Source: CAD feature listing. Evaluate the final solid. Frame: model axes, mm. Face numbers are marked on the shaded views. A direction names the side the tool comes from. Coordinates: 2 decimals unless noted, no trailing zeros. Write each loop counter-clockwise with the first axis right and the second up, starting at its lowest first coordinate (ties: lowest second). Pieces come first, ordered by that corner, then holes. Notation, with made-up numbers: (16.25, -39.5) - (48.25, -39.5) arc R17 cw to (48.25, -33.5) - close; hole circle Ø10 at (-22.75, -40). An arc over 180 degrees is marked (long way). One line per question, with ' | ' between items. Start each with the question number.
Q1. Access query for the marked faces 4 and 5. Directions: +Z, -Z, +X, -X, +Y, -Y. A direction counts if a zero-diameter tool reaches every point of the face in a straight line with its end or side. Return the directions, or none.
Q2. Draft query along X for the marked faces 1, 2 and 3. Return one class per face: +X half, -X half, draft (parallel to the pull), parting line (faces both ways), or undercut.
Q3. Cut plane A-A, the plane z = 3.2. Return loops of the section in (x, y) (3 decimals), plus the area to 3 significant figures.
Q4. Line query: line 1 (X direction, y = -63.15, z = 3.2); line 2 (Z direction, x = -11, y = -63.25); line 3 (Y direction, x = 0, z = 5.75). Output: solid intervals per line, ascending.
Q5. Cut plane C-C, the plane z = 5.5. Return loops of the section in (x, y) (3 decimals), plus the area to 3 significant figures.
Q6. Cut plane B-B, the plane x = -10.5. Return loops of the section in (y, z).
Q7. Contact query for flat-ended pins moving along their axis: P1, Ø2, axis at x = 5.5, z = 4.5, coming from the +Y side (3 decimals); P2, Ø3, axis at x = -10, z = 2, coming from the +Y side; P3, Ø2, axis at y = -54, z = 4, coming from the +X side. Output: stop coordinate, or through.
Q8. Cut plane D-D, the plane y = -40. Return loops of the section in (x, z), plus the area to 3 significant figures.
```python
from build123d import *

# Parameters (mm, degrees)
BOSS_EXTRUDE1_DEPTH = 6
SKETCH2_R           = 1.6
CUT_EXTRUDE1_DEPTH  = 10
FILLET1_R           = 1


with BuildPart() as part:
    # Sketch1 → Boss-Extrude1 (new body)
    with BuildSketch(Plane.XY):
        with BuildLine():
            Line((-6.342263295, -37.122659043), (-7.672233378, -62.5))
            Line((-7.672233378, -62.5), (-14, -62.5))
            Line((-14, -62.5), (-14, -65.5))
            Line((-14, -65.5), (14, -65.5))
            Line((14, -65.5), (14, -62.5))
            Line((14, -62.5), (7.672233378, -62.5))
            Line((7.672233378, -62.5), (6.342263295, -37.122659043))
            ThreePointArc((6.342263295, -37.122659043), (5.670701308, -36.229994036), (4.591009287, -36.516544999))
            ThreePointArc((4.591009287, -36.516544999), (0, -38.6), (-4.591009287, -36.516544999))
            ThreePointArc((-4.591009287, -36.516544999), (-5.670701308, -36.229994036), (-6.342263295, -37.122659043))
        make_face()
    extrude(amount=BOSS_EXTRUDE1_DEPTH)

    # Sketch2 → Cut-Extrude1 (cut)
    with BuildSketch(Plane.XZ.offset(65.5)):
        with Locations(Location((10.872233378, 3.2, 0), (0, 0, 270))):
            Circle(SKETCH2_R)
        with Locations(Location((-10.872233378, 3.2, 0), (0, 0, 270))):
            Circle(SKETCH2_R)
    extrude(amount=-CUT_EXTRUDE1_DEPTH, mode=Mode.SUBTRACT)

    # Fillet1
    fillet1_edges = [part.edges().sort_by_distance(p)[0] for p in [
        (-14, -64, 6),
        (14, -64, 6),
    ]]
    fillet(fillet1_edges, radius=FILLET1_R)


solid = part.part
```
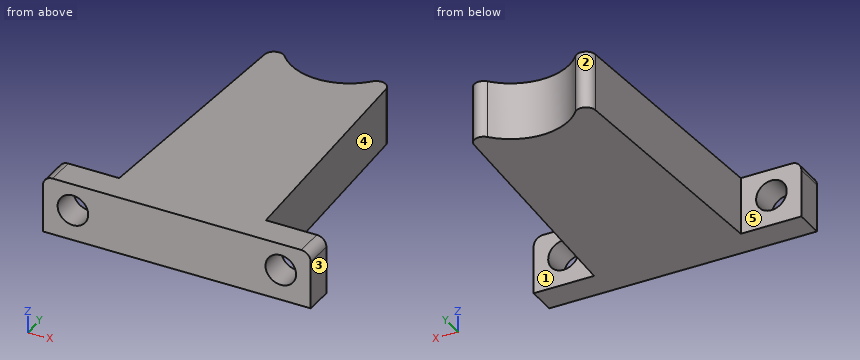
Reply:
1) face 4: +Z, -Z, +X, +Y | face 5: +Z, -Z, -X, +Y
2) face 1: draft | face 2: undercut | face 3: +X half
3) outline: (-14, -65.5) - (-12.472, -65.5) - (-12.472, -62.5) - (-14, -62.5) - close; (-9.272, -65.5) - (9.272, -65.5) - (9.272, -62.5) - (7.672, -62.5) - (6.342, -37.123) arc R1 ccw to (4.591, -36.517) arc R6.1 cw to (-4.591, -36.517) arc R1 ccw to (-6.342, -37.123) - (-7.672, -62.5) - (-9.272, -62.5) - close; (12.472, -65.5) - (14, -65.5) - (14, -62.5) - (12.472, -62.5) - close | area: 415 mm^2
4) line 1: x = -14 to -12.47, -9.27 to 9.27, 12.47 to 14 | line 2: z = 0 to 1.61, 4.79 to 6 | line 3: y = -65.5 to -38.6
5) outline: (-13.866, -65.5) - (13.866, -65.5) - (13.866, -62.5) - (7.672, -62.5) - (6.342, -37.123) arc R1 ccw to (4.591, -36.517) arc R6.1 cw to (-4.591, -36.517) arc R1 ccw to (-6.342, -37.123) - (-7.672, -62.5) - (-13.866, -62.5) - close | area: 434 mm^2
6) outline: (-65.5, 0) - (-62.5, 0) - (-62.5, 1.64) - (-65.5, 1.64) - close; (-65.5, 4.76) - (-62.5, 4.76) - (-62.5, 6) - (-65.5, 6) - close
7) P1: stops at y = -36.175 | P2: stops at y = -62.5 | P3: stops at x = 7.28
8) outline: (-6.49, 0) - (6.49, 0) - (6.49, 6) - (-6.49, 6) - close | area: 77.9 mm^2
